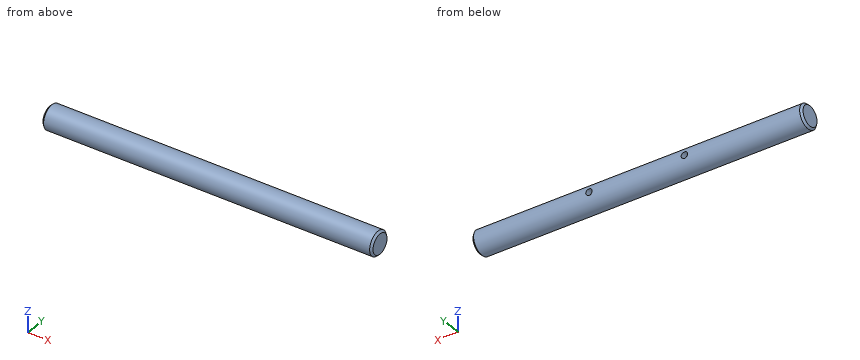
```python
from build123d import *

# Parameters (mm, degrees)
SKETCH_1_W                  = 830
SKETCH_1_H                  = 30
CHAMFER_1_SIZE              = 5
HOLE_WIZARD_16_0_16_1_D     = 16
HOLE_WIZARD_16_0_16_1_DEPTH = 15
HOLE_WIZARD_16_0_16_1_TIP   = 4.806884952


with BuildPart() as part:
    # 草图1 → 旋转1 (revolve)
    with BuildSketch(Plane.XY):
        with Locations((-415, 15)):
            Rectangle(SKETCH_1_W, SKETCH_1_H)
    revolve(axis=Axis((0, 0, 0), (-1, 0, 0)))

    # 倒角1
    chamfer_1_edges = [part.edges().sort_by_distance(p)[0] for p in [
        (0, -30, 0),
        (-830, -30, 0),
    ]]
    chamfer(chamfer_1_edges, length=CHAMFER_1_SIZE)

    # Ø16.0 (16) 直径孔1
    with Locations(Plane(origin=(0, 30, 0), x_dir=(1, 0, 0), z_dir=(0, 1, 0))):
        with Locations((-535, 0), (-295, 0)):
            Hole(HOLE_WIZARD_16_0_16_1_D / 2, depth=HOLE_WIZARD_16_0_16_1_DEPTH)
            with Locations((0, 0, -(HOLE_WIZARD_16_0_16_1_DEPTH + HOLE_WIZARD_16_0_16_1_TIP / 2))):  # 118° drill point
                Cone(0, HOLE_WIZARD_16_0_16_1_D / 2, HOLE_WIZARD_16_0_16_1_TIP, mode=Mode.SUBTRACT)


solid = part.part
```
CAD build for the part. Positions are in the model's coordinates, mm. Coordinates: 2 decimals unless noted, no trailing zeros. Write each loop counter-clockwise with the first axis right and the second up, starting at its lowest first coordinate (ties: lowest second). Pieces come first, ordered by that corner, then holes.
(1) Cut at A-A, the plane x = -144.5. List the corners of the cut face in (y, z).
(2) Flat gauge pins, fed straight in: pin 1 (10 mm diameter, centred on x = -546, z = 6.5, fed in from -Y); pin 2 (6 mm diameter, centred on x = -225.5, y = -19, fed in from +Z); pin 3 (2 mm diameter, centred on x = -592, y = -23.5, fed in from -Z). Where does each tip first touch, or does it go through?
(3) Drill centre lines: probe 1 along Y at (x, z) = (-366, -1); probe 2 along X at (y, z) = (20, 7); probe 3 along Z at (x, y) = (-295, 23.5). Where is each one in solid material? Low to high.
Geometry says:
1. outline: circle Ø60 at (0, 0)
2. pin 1: stops at y = -29.96
2. pin 2: stops at z = 25.38
2. pin 3: stops at z = -19.84
3. probe 1: y = -29.98 to 29.98
3. probe 2: x = -830 to -538.87, -531.13 to -298.87, -291.13 to 0
3. probe 3: z = -18.65 to -8, 8 to 18.65
